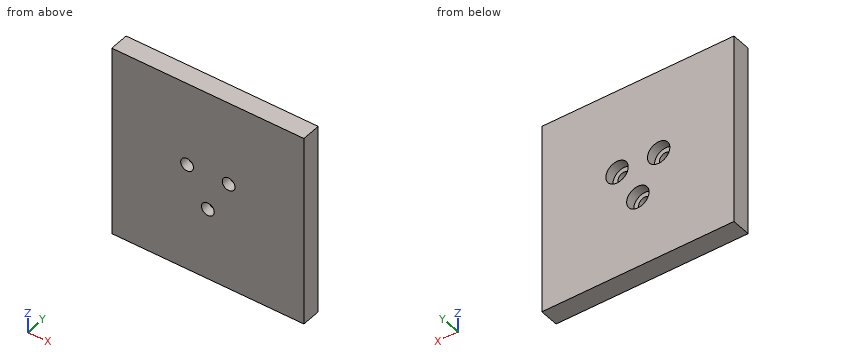
from build123d import *

# Parameters (mm, degrees)
SKETCH1_W           = 60
SKETCH1_H           = 60
BOSS_EXTRUDE2_DEPTH = 6
SKETCH1_4_R         = 2
CUT_EXTRUDE1_DEPTH  = 7
CUT_EXTRUDE2_START  = 6
SKETCH1_5_R         = 3.5
CUT_EXTRUDE2_DEPTH  = 3


with BuildPart() as part:
    # Sketch1 → Boss-Extrude2 (new body)
    with BuildSketch(Plane(origin=(0, 0, 0), x_dir=(1, 0, 0), z_dir=(0, 1, 0))):
        Rectangle(SKETCH1_W, SKETCH1_H)
    extrude(amount=BOSS_EXTRUDE2_DEPTH)

    # Sketch1<4> → Cut-Extrude1 (cut, through all)
    with BuildSketch(Plane(origin=(0, 0, 0), x_dir=(1, 0, 0), z_dir=(0, 1, 0))):
        with Locations((0, 7.5)):
            Circle(SKETCH1_4_R)
        with Locations((6.495190528, -3.75)):
            Circle(SKETCH1_4_R)
        with Locations((-6.495190528, -3.75)):
            Circle(SKETCH1_4_R)
    extrude(amount=CUT_EXTRUDE1_DEPTH, mode=Mode.SUBTRACT)

    # Sketch1<5> → Cut-Extrude2 (cut)
    with BuildSketch(Plane(origin=(0, 0, 0), x_dir=(1, 0, 0), z_dir=(0, 1, 0)).offset(CUT_EXTRUDE2_START)):
        with Locations((0, 7.5)):
            Circle(SKETCH1_5_R)
        with Locations((6.495190528, -3.75)):
            Circle(SKETCH1_5_R)
        with Locations((-6.495190528, -3.75)):
            Circle(SKETCH1_5_R)
    extrude(amount=-CUT_EXTRUDE2_DEPTH, mode=Mode.SUBTRACT)


solid = part.part
Work out the finished part from the listing and answer in its coordinate system (mm). Give positions to 0.01 mm unless a question says otherwise; leave off trailing zeros. Order: outer loops, then holes, each group sorted by start corner. A loop starts at its lowest first (then second) coordinate and runs counter-clockwise, first axis right, second up. Notation, with made-up numbers: (-23.75, 40.5) -> (20.25, 40.5) arc R37 cw to (20.25, 79.5) -> close; hole circle Ø6 at (-6, 69). An arc over 180 degrees is marked (long way). Answer as a JSON object with one key per item and string values. Group by question number.
1. A flat-ended cylindrical pin translates along its axis: pin 1 Ø5 at (x, z) = (6.5, 3.75) entering from +Y. Find the tip coordinate at first contact, or state that the pin passes through.
2. Section C-C on y = 3.75 is taken. Determine the outline of the cut face in (x, z).
3. Section B-B on z = -7.5 is taken. Determine the outline of the cut face in (x, y).
4. Section D-D on z = 3.75 is taken. Determine the outline of the cut face in (x, y), plus the area to 3 significant figures.
5. Section A-A on x = 0 is taken. Determine the outline of the cut face in (y, z).
6. Consider line 1 along X through (y, z) = (1.35, 3.75); line 2 along Z through (x, y) = (0, 4.35); line 3 along X through (y, z) = (4.2, 3.75). Determine where each line is inside the solid, lowest interval first. Write a range as [from, to].
Result sheet:
{
 "1": {"pin 1": "stops at y = 3"},
 "2": {"outline": "(-30, -30) -> (30, -30) -> (30, 30) -> (-30, 30) -> close; hole circle Ø7 at (-6.5, 3.75); hole circle Ø7 at (0, -7.5); hole circle Ø7 at (6.5, 3.75)"},
 "3": {"outline": "(-30, 0) -> (-2, 0) -> (-2, 3) -> (-3.5, 3) -> (-3.5, 6) -> (-30, 6) -> close; (2, 0) -> (30, 0) -> (30, 6) -> (3.5, 6) -> (3.5, 3) -> (2, 3) -> close"},
 "4": {"outline": "(-30, 0) -> (-8.5, 0) -> (-8.5, 3) -> (-10, 3) -> (-10, 6) -> (-30, 6) -> close; (-4.5, 0) -> (4.5, 0) -> (4.5, 3) -> (3, 3) -> (3, 6) -> (-3, 6) -> (-3, 3) -> (-4.5, 3) -> close; (8.5, 0) -> (30, 0) -> (30, 6) -> (10, 6) -> (10, 3) -> (8.5, 3) -> close", "area": "294 mm^2"},
 "5": {"outline": "(0, -30) -> (6, -30) -> (6, -11) -> (3, -11) -> (3, -9.5) -> (0, -9.5) -> close; (0, -5.5) -> (3, -5.5) -> (3, -4) -> (6, -4) -> (6, 30) -> (0, 30) -> close"},
 "6": {"line 1": "x = [-30, -8.5], [-4.5, 4.5], [8.5, 30]", "line 2": "z = [-30, -11], [-4, 30]", "line 3": "x = [-30, -10], [-3, 3], [10, 30]"}
}
